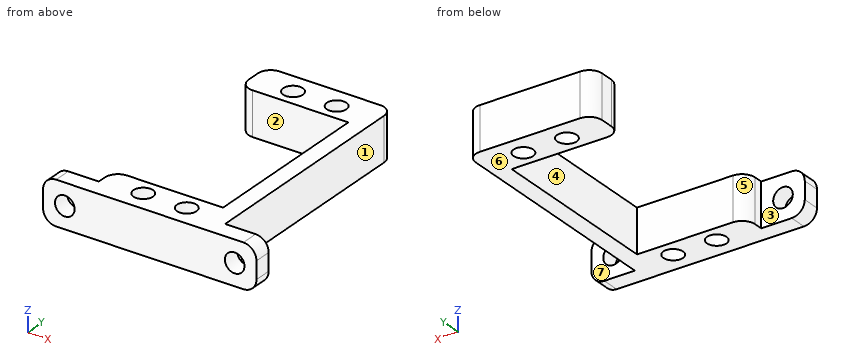
```python
from build123d import *

# Parameters (mm, degrees)
SKETCH_1_W          = 10
SKETCH_1_H          = 4
SKETCH_1_R          = 2.25
EXTRUDE_1_DEPTH     = 10
SKETCH_2_R          = 2.25
CUT_EXTRUDE_1_DEPTH = 10
FILLET_1_R          = 3


with BuildPart() as part:
    # 草图1 → 凸台-拉伸1 (new body)
    with BuildSketch(Plane.XY):
        with Locations((-19.5, -27.5)):
            Rectangle(SKETCH_1_W, SKETCH_1_H)
        Polygon((-14.5, -20.5), (-10.5, -20.5), (10.5, -20.5), (10.5, 20.5), (-10.5, 20.5), (-14.5, 20.5), (-14.5, 29.5), (14.5, 29.5), (14.5, -29.5), (-14.5, -29.5), align=None)
        with Locations((5, 24.5)):
            Circle(SKETCH_1_R, mode=Mode.SUBTRACT)
        with Locations((-5, 24.5)):
            Circle(SKETCH_1_R, mode=Mode.SUBTRACT)
        with Locations((5, -24.5)):
            Circle(SKETCH_1_R, mode=Mode.SUBTRACT)
        with Locations((-5, -24.5)):
            Circle(SKETCH_1_R, mode=Mode.SUBTRACT)
        with Locations((19.5, -27.5)):
            Rectangle(SKETCH_1_W, SKETCH_1_H)
    extrude(amount=EXTRUDE_1_DEPTH)

    # 草图2 → 切除-拉伸1 (cut)
    with BuildSketch(Plane(origin=(0, -25.5, 0), x_dir=(1, 0, 0), z_dir=(0, 1, 0))):
        with Locations((19.5, -5)):
            Circle(SKETCH_2_R)
        with Locations((-19.5, -5)):
            Circle(SKETCH_2_R)
    extrude(amount=-CUT_EXTRUDE_1_DEPTH, mode=Mode.SUBTRACT)

    # 圆角1
    fillet_1_edges = [part.edges().sort_by_distance(p)[0] for p in [
        (-24.5, -27.5, 10),
        (24.5, -27.5, 0),
        (24.5, -27.5, 10),
        (-24.5, -27.5, 0),
        (-14.5, -20.5, 5),
        (-14.5, 20.5, 5),
        (-14.5, 29.5, 5),
        (14.5, 29.5, 5),
    ]]
    fillet(fillet_1_edges, radius=FILLET_1_R)


solid = part.part
```
Input: part model. Units: mm. Frame: model coordinates. Face numbers are marked on the shaded views. A direction names the side the tool comes from. Round coordinates to 2 decimals unless told otherwise and drop trailing zeros. Write each loop counter-clockwise with the first axis right and the second up, starting at its lowest first coordinate (ties: lowest second). Pieces come first, ordered by that corner, then holes. Notation, with made-up numbers: (40, 27) -> (54, 27) arc R21 ccw to (54, 57) -> close; hole circle Ø1 at (20, -21). An arc over 180 degrees is marked (long way). Answer as CSV lines item,"result".
1. Contact query for flat-ended pins moving along their axis: P1, Ø5, axis at x = 20.5, z = 7.5, coming from the +Y side; P2, Ø1, axis at y = 7.5, z = 7.5, coming from the +X side; P3, Ø1, axis at y = -19, z = 4.5, coming from the -X side. Output: stop coordinate, or through.
Geometry says:
P1,"stops at y = -25.5"
P2,"stops at x = 14.5"
P3,"stops at x = 10.5"
2. Reachability of the marked faces 1, 2 and 3 from +Z, -Z, +X, -X, +Y, -Y: full face, straight path, thin tool, end or side. Return the list, or none.
Geometry says:
face 1,"+Z, -Z, +X, +Y"
face 2,"+Z, -Z, -X"
face 3,"+Z, -Z, -X, +Y"
3. Section A-A (z = 5). Return the cut outline in (x, y), plus the area to 3 significant figures.
Geometry says:
outline,"(-24.5, -29.5) -> (-21.75, -29.5) -> (-21.75, -25.5) -> (-24.5, -25.5) -> close; (-17.25, -29.5) -> (17.25, -29.5) -> (17.25, -25.5) -> (14.5, -25.5) -> (14.5, 26.5) arc R3 ccw to (11.5, 29.5) -> (-11.5, 29.5) arc R3 ccw to (-14.5, 26.5) -> (-14.5, 23.5) arc R3 ccw to (-11.5, 20.5) -> (10.5, 20.5) -> (10.5, -20.5) -> (-11.5, -20.5) arc R3 ccw to (-14.5, -23.5) -> (-14.5, -25.5) -> (-17.25, -25.5) -> close; (21.75, -29.5) -> (24.5, -29.5) -> (24.5, -25.5) -> (21.75, -25.5) -> close; hole circle Ø4.5 at (-5, -24.5); hole circle Ø4.5 at (-5, 24.5); hole circle Ø4.5 at (5, -24.5); hole circle Ø4.5 at (5, 24.5)"
area,"659 mm^2"
4. Ray query, L1, parallel to X at y = -27.6, z = 5; L2, parallel to Y at x = 5, z = 7.5; L3, parallel to Y at x = -8, z = 3.5. Return the intervals inside material, ascending. Write a range as [from, to].
Geometry says:
L1,"x = [-24.5, -21.75], [-17.25, 17.25], [21.75, 24.5]"
L2,"y = [-29.5, -26.75], [-22.25, -20.5], [20.5, 22.25], [26.75, 29.5]"
L3,"y = [-29.5, -20.5], [20.5, 29.5]"
5. Section D-D (x = -5). Return the cut outline in (y, z).
Geometry says:
outline,"(-29.5, 0) -> (-26.75, 0) -> (-26.75, 10) -> (-29.5, 10) -> close; (-22.25, 0) -> (-20.5, 0) -> (-20.5, 10) -> (-22.25, 10) -> close; (20.5, 0) -> (22.25, 0) -> (22.25, 10) -> (20.5, 10) -> close; (26.75, 0) -> (29.5, 0) -> (29.5, 10) -> (26.75, 10) -> close"
6. Section C-C (y = 24.5). Return the cut outline in (x, z).
Geometry says:
outline,"(-14.5, 0) -> (-7.25, 0) -> (-7.25, 10) -> (-14.5, 10) -> close; (-2.75, 0) -> (2.75, 0) -> (2.75, 10) -> (-2.75, 10) -> close; (7.25, 0) -> (14.5, 0) -> (14.5, 10) -> (7.25, 10) -> close"
7. Mould query, pull axis Y, two halves, no side actions, for the marked faces 4, 5, 6 and 7. Classes: +Y half, -Y half, draft (parallel to the pull), parting line (faces both ways), or undercut.
Geometry says:
face 4,"undercut"
face 5,"undercut"
face 6,"draft"
face 7,"+Y half"
8. Section B-B (x = 9). Return the cut outline in (y, z), plus the area to 3 significant figures.
Geometry says:
outline,"(-29.5, 0) -> (-20.5, 0) -> (-20.5, 10) -> (-29.5, 10) -> close; (20.5, 0) -> (29.5, 0) -> (29.5, 10) -> (20.5, 10) -> close"
area,"180 mm^2"
